from build123d import *

# Parameters (mm, degrees)
F0_W     = 90.549692
F0_H     = 75.335876
F1_DEPTH = 25.4
F2_R     = 25.4
F3_T     = -2.54


with BuildPart() as f1:
    # F0 (on Front) → F1 (new body)
    with BuildSketch(Plane.XZ):
        Rectangle(F0_W, F0_H)
    extrude(amount=-F1_DEPTH)

    # F2
    f2_edges = [f1.edges().sort_by_distance(p)[0] for p in [
        (45.274846, 12.7, 37.667938),
    ]]
    fillet(f2_edges, radius=F2_R)

    # F3
    f3_openings = [f1.faces().sort_by_distance(p)[0] for p in [
        (-0.820402, 0, -0.662813),
    ]]
    offset(amount=F3_T, openings=f3_openings)


solid = f1.part
Could you check a few things on this model? Use its own coordinates, in mm. A direction names the side the tool comes from. Give positions to 0.01 mm unless a question says otherwise; leave off trailing zeros. Order: outer loops, then holes, each group sorted by start corner. A loop starts at its lowest first (then second) coordinate and runs counter-clockwise, first axis right, second up. Notation, with made-up numbers: (-27.5, 52) -> (-2.5, 52) arc R21 ccw to (-2.5, 86) -> close; hole circle Ø8 at (18.5, 83). An arc over 180 degrees is marked (long way). Answer in a Markdown table with one row per item. Add a question column.
Item 1: Imagine slicing it at A-A (x = 8). List the corners of the cut face in (y, z) for me.
Item 2: I'm going to push a flat-ended pin straight in: P1, Ø1, axis at x = 17.5, z = -29, coming from the -Y side. Where does the tip first touch, or does it pass through?
Item 3: Please list where these lines run through material, in increasing order: probe 1 along Z at (x, y) = (-27.5, 18); probe 2 along X at (y, z) = (16.5, -20.5); probe 3 along Y at (x, z) = (-33, -14).
Item 4: We'd pull the mould along Z, two halves only. Please class faces 1 (the flat face through (-13, 13, 37.668)), 2 (the flat face through (42.735, 11, -12)), 3 (the flat face through (-1, 13, -37.668)), 4 (the flat face through (45.275, 13, -13)): pulls with the +Z half, pulls with the -Z half, needs draft (parallel to the pull), parting line crosses it, or undercut.
Item 5: For faces 5 (the flat face through (-1, 25.4, 1)), 6 (the flat face through (-42.735, 11, 0)), which set-ups out of +Z, -Z, +X, -X, +Y, -Y let a thin tool reach every point of the face, with its end or its side?
Item 6: Imagine slicing it at B-B (y = 14.25). List the corners of the cut face in (x, z) for me.
Item 7: Imagine slicing it at C-C (z = -14). List the corners of the cut face in (x, y) for me.
Result:
| question | item | result |
|---|---|---|
| 1 | outline | (0, -37.67) -> (25.4, -37.67) -> (25.4, 37.67) -> (0, 37.67) -> (0, 35.13) -> (22.86, 35.13) -> (22.86, -35.13) -> (0, -35.13) -> close |
| 2 | P1 | y = 22.86 |
| 3 | probe 1 | -37.67 to -35.13, 35.13 to 37.67 |
| 3 | probe 2 | -45.27 to -42.73, 42.73 to 45.27 |
| 3 | probe 3 | 22.86 to 25.4 |
| 4 | face 1 | pulls with the +Z half |
| 4 | face 2 | undercut |
| 4 | face 3 | pulls with the -Z half |
| 4 | face 4 | needs draft |
| 5 | face 5 | +Z, -Z, +X, -X, +Y |
| 5 | face 6 | -Y |
| 6 | outline | (-45.27, -37.67) -> (45.27, -37.67) -> (45.27, 12.27) arc R25.4 ccw to (19.87, 37.67) -> (-45.27, 37.67) -> close; hole (-42.73, -35.13) -> (42.73, -35.13) -> (42.73, 12.27) arc R22.86 ccw to (19.87, 35.13) -> (-42.73, 35.13) -> close |
| 7 | outline | (-45.27, 0) -> (-42.73, 0) -> (-42.73, 22.86) -> (42.73, 22.86) -> (42.73, 0) -> (45.27, 0) -> (45.27, 25.4) -> (-45.27, 25.4) -> close |
